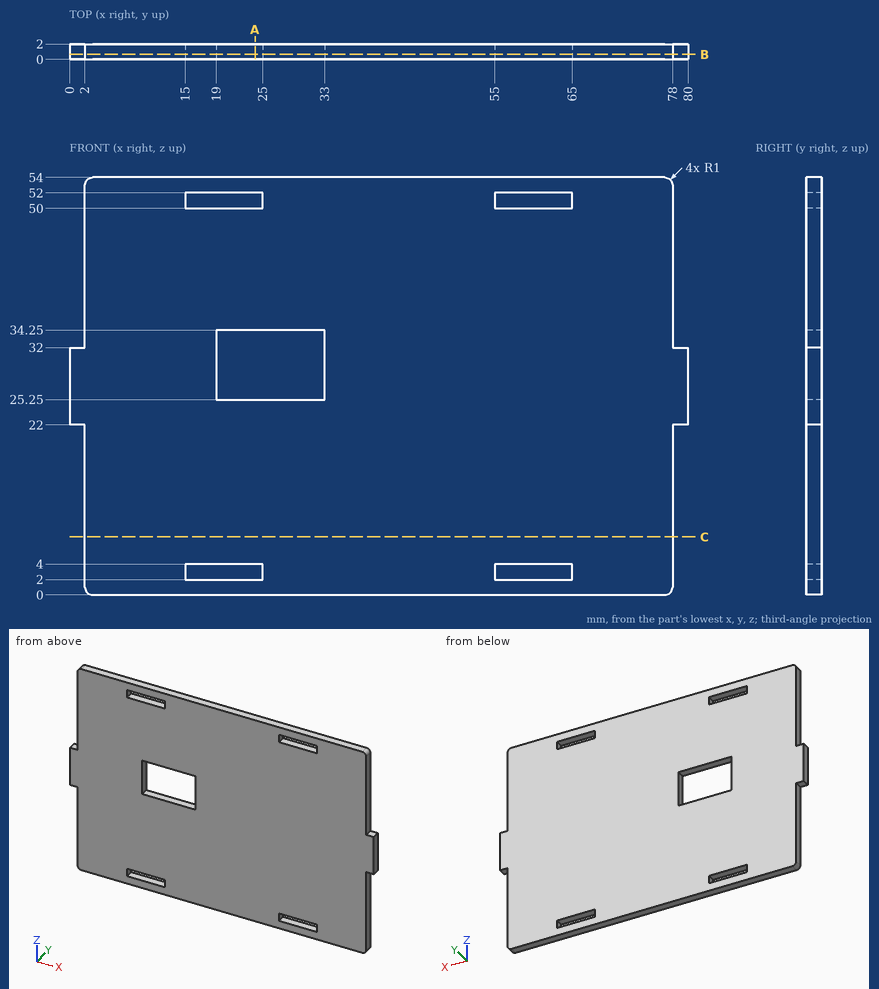
Verification items for this drawing (mm, ordinates from the low corner). Round coordinates to 2 decimals unless told otherwise and drop trailing zeros. Loops run counter-clockwise (first coordinate to the right, second up) from the corner with the lowest first, then second, coordinate; pieces in that order, holes last. Notation, with made-up numbers: M 49.5,88 L 63.5,88 A18 cw 63.5,112 Z; hole C 65.5,82 d5. An arc over 180 degrees is marked long. Answer as a JSON object with one key per item and string values.
1. Gauge pin test, flat ends, axial feed: P1, Ø1, axis at y = 1, z = 10, coming from the -X side; P2, Ø0.6, axis at x = 78.5, y = 0.5, coming from the +Z side. Record the tip position at first contact, or that the pin passes through.
Reply:
{"P1": "stops at x = 2", "P2": "stops at z = 32"}
2. Section check C-C (z = 7.5). Record the boundary of the cut face in (x, y).
Reply:
{"outline": "M 2,0 L 78,0 L 78,2 L 2,2 Z"}
3. Section check A-A (x = 24). Record the boundary of the cut face in (y, z), plus the area to 3 significant figures.
Reply:
{"outline": "M 0,0 L 2,0 L 2,2 L 0,2 Z; M 0,4 L 2,4 L 2,25.25 L 0,25.25 Z; M 0,34.25 L 2,34.25 L 2,50 L 0,50 Z; M 0,52 L 2,52 L 2,54 L 0,54 Z", "area": "82.0 mm²"}
4. Scan lines: line 1 (Z direction, x = 60, y = 1.3); line 2 (Z direction, x = 23, y = 1.65); line 3 (X direction, y = 0.95, z = 26). Record each from-to range of solid material in increasing order.
Reply:
{"line 1": "z = 0 to 2, 4 to 50, 52 to 54", "line 2": "z = 0 to 2, 4 to 25.25, 34.25 to 50, 52 to 54", "line 3": "x = 0 to 19, 33 to 80"}
5. Section check B-B (y = 0.65). State how many separate pieces and enclosed holes the cut face has, plus the area to 3 significant figures.
Reply:
{"separate pieces": "1", "enclosed holes": "5", "area": "3,940 mm²"}
